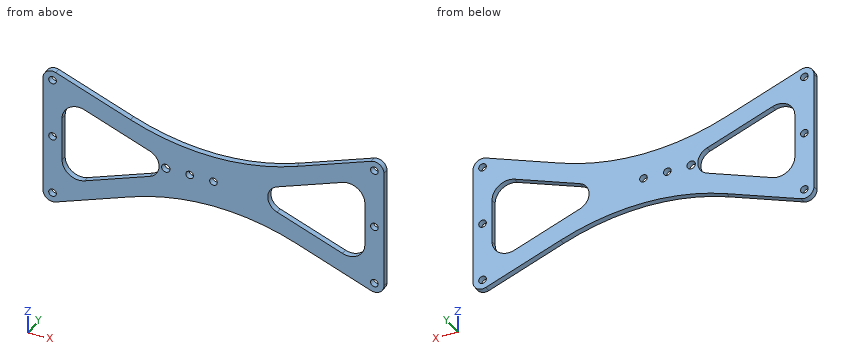
from build123d import *

# Parameters (mm, degrees)
SKETCH1_R           = 2.032
BOSS_EXTRUDE1_DEPTH = 3.175
FILLET1_R           = 8.89
FILLET2_R           = 7.62
FILLET3_R           = 127
SKETCH1_3_R         = 2.032
SKETCH1_3_R_2       = 2.2225
CUT_EXTRUDE1_DEPTH  = 99.041203328


with BuildPart() as part:
    # Sketch1 → Boss-Extrude1 (new body)
    with BuildSketch(Plane(origin=(0, 0, 0), x_dir=(1, 0, 0), z_dir=(0, 1, 0))):
        with BuildLine():
            Line((0, -5.417229233), (83.960643072, -36.513763704))
            ThreePointArc((83.960643072, -36.513763704), (88.627022296, -35.919492367), (90.805, -31.75))
            Line((90.805, -31.75), (90.805, 31.75))
            ThreePointArc((90.805, 31.75), (88.627022296, 35.919492367), (83.960643072, 36.513763704))
            Line((83.960643072, 36.513763704), (0, 5.417229233))
            Line((0, 5.417229233), (-83.960643072, 36.513763704))
            ThreePointArc((-83.960643072, 36.513763704), (-88.627022296, 35.919492367), (-90.805, 31.75))
            Line((-90.805, 31.75), (-90.805, -31.75))
            ThreePointArc((-90.805, -31.75), (-88.627022296, -35.919492367), (-83.960643072, -36.513763704))
            Line((-83.960643072, -36.513763704), (0, -5.417229233))
        make_face()
        Polygon((-80.645, 24.451289285), (-14.62651893, 0), (-80.645, -24.451289285), align=None, mode=Mode.SUBTRACT)
        Polygon((80.645, -24.451289285), (14.62651893, 0), (80.645, 24.451289285), align=None, mode=Mode.SUBTRACT)
        with Locations(Location((85.725, 0, 0), (0, 0, 270))):
            Circle(SKETCH1_R, mode=Mode.SUBTRACT)
        with Locations(Location((85.725, 31.75, 0), (0, 0, 270))):
            Circle(SKETCH1_R, mode=Mode.SUBTRACT)
        with Locations(Location((85.725, -31.75, 0), (0, 0, 270))):
            Circle(SKETCH1_R, mode=Mode.SUBTRACT)
        with Locations(Location((-85.725, -31.75, 0), (0, 0, 270))):
            Circle(SKETCH1_R, mode=Mode.SUBTRACT)
        with Locations(Location((-85.725, 31.75, 0), (0, 0, 270))):
            Circle(SKETCH1_R, mode=Mode.SUBTRACT)
        with Locations(Location((-85.725, 0, 0), (0, 0, 270))):
            Circle(SKETCH1_R, mode=Mode.SUBTRACT)
    extrude(amount=BOSS_EXTRUDE1_DEPTH)

    # Fillet1
    fillet1_edges = [part.edges().sort_by_distance(p)[0] for p in [
        (80.645, 1.5875, -24.451289285),
        (80.645, 1.5875, 24.451289285),
        (-80.645, 1.5875, -24.451289285),
        (-80.645, 1.5875, 24.451289285),
    ]]
    fillet(fillet1_edges, radius=FILLET1_R)

    # Fillet2
    fillet2_edges = [part.edges().sort_by_distance(p)[0] for p in [
        (14.62651893, 1.5875, 0),
        (-14.62651893, 1.5875, 0),
    ]]
    fillet(fillet2_edges, radius=FILLET2_R)

    # Fillet3
    fillet3_edges = [part.edges().sort_by_distance(p)[0] for p in [
        (0, 1.5875, 5.417229233),
        (0, 1.5875, -5.417229233),
    ]]
    fillet(fillet3_edges, radius=FILLET3_R)

    # Sketch1_3 → Cut-Extrude1 (cut, through all)
    with BuildSketch(Plane(origin=(0, 0, 0), x_dir=(1, 0, 0), z_dir=(0, 1, 0))):
        with Locations(Location((0, 0, 0), (0, 0, 270))):
            Circle(SKETCH1_3_R)
        with Locations(Location((-12.7, 0, 0), (0, 0, 270))):
            Circle(SKETCH1_3_R)
        with Locations(Location((-25.4, 0, 0), (0, 0, 270))):
            Circle(SKETCH1_3_R_2)
    extrude(amount=CUT_EXTRUDE1_DEPTH, mode=Mode.SUBTRACT)


solid = part.part
Input: part model. Units: mm. Frame: model coordinates. Give positions to 0.01 mm unless a question says otherwise; leave off trailing zeros. Order: outer loops, then holes, each group sorted by start corner. A loop starts at its lowest first (then second) coordinate and runs counter-clockwise, first axis right, second up. Notation, with made-up numbers: (54, 3.5) - (68, 3.5) arc R28 cw to (68, 25.5) - close; hole circle Ø1 at (-7, 4.5). An arc over 180 degrees is marked (long way). Answer as a JSON object with one key per item and string values. Group by question number.
Q1. Cut plane B-B, the plane x = -25.4. Output: boundary loops of the cut face in (y, z) (1 decimal), then the cut area to 3 significant figures.
Q2. Cut plane A-A, the plane z = 0. Count the separate pieces of the cut face and the enclosed holes in it, then the cut area to 3 significant figures.
Q3. Line query: probe 1 along X at (y, z) = (2.35, -3) (3 decimals); probe 2 along X at (y, z) = (1.25, 2.5) (3 decimals); probe 3 along Z at (x, y) = (72, 1.4). Output: solid intervals per line, ascending.
Q4. Cut plane C-C, the plane z = 26. Output: boundary loops of the cut face in (x, y) (3 decimals).
Q5. First-contact query: pin 1 Ø2.5 at (x, z) = (85.725, -31.75) entering from -Y (3 decimals); pin 2 Ø1 at (x, y) = (39.5, 2.5) entering from +Z. Flat tips, straight axial feed; report the tip coordinate or a pass-through.
Results:
{
 "1": {"outline": "(0, -16.4) - (3.2, -16.4) - (3.2, -2.2) - (0, -2.2) - close; (0, 2.2) - (3.2, 2.2) - (3.2, 16.4) - (0, 16.4) - close", "area": "90.1 mm^2"},
 "2": {"separate pieces": "8", "enclosed holes": "0", "area": "183 mm^2"},
 "3": {"probe 1": "-90.805 to -80.645, -29.562 to 29.562, 80.645 to 90.805", "probe 2": "-90.805 to -80.645, -29.368 to 29.368, 80.645 to 90.805", "probe 3": "-32.08 to -20.57, 20.57 to 32.08"},
 "4": {"outline": "(-90.805, 0) - (-55.573, 0) - (-55.573, 3.175) - (-90.805, 3.175) - close; (55.573, 0) - (90.805, 0) - (90.805, 3.175) - (55.573, 3.175) - close"},
 "5": {"pin 1": "through", "pin 2": "z = 20.31"}
}
